Source: CAD feature listing. Evaluate the final solid. Frame: model axes, mm. Give positions to 0.01 mm unless a question says otherwise; leave off trailing zeros. Order: outer loops, then holes, each group sorted by start corner. A loop starts at its lowest first (then second) coordinate and runs counter-clockwise, first axis right, second up.
from build123d import *

# Parameters (mm, degrees)
F0_W     = 101.6
F0_H     = 177.8
F0_R     = 1.5875
F1_DEPTH = 3.175
F3_DEPTH = 25.4
F5_DEPTH = 3.175


with BuildPart() as f1:
    # F0 (on Top) → F1 (new body)
    with BuildSketch(Plane.XY):
        with Locations((50.8, 88.9)):
            Rectangle(F0_W, F0_H)
        with Locations((19.05, 15.875)):
            Circle(F0_R, mode=Mode.SUBTRACT)
        with Locations((50.897908, 31.750108)):
            Circle(F0_R, mode=Mode.SUBTRACT)
        with Locations((82.728313, 15.910065)):
            Circle(F0_R, mode=Mode.SUBTRACT)
        with Locations((50.897908, 76.200108)):
            Circle(F0_R, mode=Mode.SUBTRACT)
        with Locations((50.8, 120.65)):
            Circle(F0_R, mode=Mode.SUBTRACT)
        with Locations((19.05, 160.3375)):
            Circle(F0_R, mode=Mode.SUBTRACT)
        with Locations((82.569213, 160.372478)):
            Circle(F0_R, mode=Mode.SUBTRACT)
    extrude(amount=F1_DEPTH)

    # F2 (on face) → F3 (cut)
    with BuildSketch(Plane.XY.offset(3.175)):
        with BuildLine():
            Line((101.6, 0), (101.6, 177.8))
            ThreePointArc((101.6, 177.8), (77.779317, 88.9), (101.6, 0))
        make_face()
        with BuildLine():
            ThreePointArc((0, 0), (23.820683, 88.9), (0, 177.8))
            Line((0, 177.8), (0, 0))
        make_face()
    extrude(amount=-F3_DEPTH, mode=Mode.SUBTRACT)

    # F4 (on face) → F5 (join, through all)
    with BuildSketch(Plane.XY.offset(3.175)):
        with BuildLine():
            Line((0, 177.8), (101.6, 177.8))
            ThreePointArc((101.6, 177.8), (50.8, 203.2), (0, 177.8))
        make_face()
        with BuildLine():
            ThreePointArc((0, 0), (50.8, -25.4), (101.6, 0))
            Line((101.6, 0), (0, 0))
        make_face()
    extrude(amount=-F5_DEPTH)


solid = f1.part
1) Section query C-C on y = 63. Output: boundary loops of the cut face in (x, z) (3 decimals).
Checks:
outline: (21.924, 0) - (79.676, 0) - (79.676, 3.175) - (21.924, 3.175) - close
2) Ray query, L1, parallel to X at y = 161, z = 2.8; L2, parallel to X at y = 120.65, z = 1.7; L3, parallel to Y at x = 50, z = 2.4. Return the intervals inside material, ascending.
Checks:
L1: x = 8.55 to 17.61, 20.49 to 81.11, 84.03 to 93.05
L2: x = 20.96 to 49.21, 52.39 to 80.64
L3: y = -25.39 to 30.44, 33.06 to 74.89, 77.51 to 119.28, 122.02 to 203.19
3) Pull-direction query (Y, two-part tool) for faces 1 (the face through (23.816, 87.597, 1.61)), 2 (the face through (49.976, -25.395, 1.61)), 3 (the face through (77.784, 90.203, 1.61)), 4 (the face through (50, 91, 0)); classes: +Y half, -Y half, draft (parallel to the pull), parting line (faces both ways), or undercut.
Checks:
face 1: undercut
face 2: -Y half
face 3: undercut
face 4: draft
4) First-contact query: pin 1 Ø1.5 at (x, z) = (47, 1.5) entering from +Y; pin 2 Ø3 at (x, y) = (19.05, 15.875) entering from -Z; pin 3 Ø1.5 at (x, z) = (71, 1.5) entering from +Y. Flat tips, straight axial feed; report the tip coordinate or a pass-through.
Checks:
pin 1: stops at y = 203.13
pin 2: passes through
pin 3: stops at y = 200.15
5) Section query A-A on z = 1.4. State how many separate pieces and enclosed holes the cut face has, and give its area (3 significant figures).
Checks:
separate pieces: 1
enclosed holes: 7
area: 15,900 mm2
6) Section query B-B on x = 33. Output: boundary loops of the cut face in (y, z) (3 decimals), and give its area (3 significant figures).
Checks:
outline: (-22.854, 0) - (200.654, 0) - (200.654, 3.175) - (-22.854, 3.175) - close
area: 710 mm2
